Check sheet for the modelled part. Datum: model origin and axes. Units: mm. Round coordinates to 2 decimals unless told otherwise and drop trailing zeros. Loops run counter-clockwise (first coordinate to the right, second up) from the corner with the lowest first, then second, coordinate; pieces in that order, holes last. Notation, with made-up numbers: (85.25, 4) - (142.25, 4) arc R8 cw to (142.25, 15) - close; hole circle Ø4 at (56.25, 74.5). An arc over 180 degrees is marked (long way). Put each result on its own line as item: value. Start each with the question number.
Item 1: Material ranges on line 1 along X through (y, z) = (6, -5); line 2 along X through (y, z) = (9, -41.5); line 3 along Y through (x, z) = (26.75, -26.5), recorded low to high.
Item 2: Section check A-A, the plane z = -11. Record the cut outline in (x, y) (3 decimals).
Item 3: Section check C-C, the plane y = 8.5. Record the cut outline in (x, z), and give its area (3 significant figures).
Item 4: Draft check along X on faces 1 (the flat face through (16, 8, -50.8)), 2 (the cylindrical face through (15.806, 18.283, -25.756)), 3 (the flat face through (25.434, 10.939, -25.044)). Enter one of: pulls with the +X half, pulls with the -X half, needs draft (parallel to the pull), parting line crosses it, or undercut.
Item 5: Gauge pin test, flat ends, axial feed: pin 1 Ø4 at (x, z) = (14, -26.5) entering from +Y; pin 2 Ø1 at (x, z) = (23, -16) entering from +Y; pin 3 Ø5 at (y, z) = (8.5, -36) entering from +X. Record the tip position at first contact, or that the pin passes through.
Item 6: Section check B-B, the plane x = 14. Record the cut outline in (y, z), and give its area (3 significant figures).
from build123d import *

# Parameters (mm, degrees)
SKETCH1_W           = 31.75
SKETCH1_H           = 19.05
BOSS_EXTRUDE1_DEPTH = 50.8
CUT_EXTRUDE1_DEPTH  = 63.861792847
CUT_EXTRUDE2_START  = -50.8
CUT_EXTRUDE2_DEPTH  = 50.8


# Read off the part's stored shape, not the designer's step: Cut-Extrude2
with BuildPart() as part:
    # Sketch1 → Boss-Extrude1 (new body)
    with BuildSketch(Plane.XY):
        with Locations((15.875, 9.525)):
            Rectangle(SKETCH1_W, SKETCH1_H)
    extrude(amount=-BOSS_EXTRUDE1_DEPTH)

    # Sketch2 → Cut-Extrude1 (cut, through all)
    with BuildSketch(Plane.XY):
        Polygon((0, 19.05), (0, 0), (10.998522628, 19.05), align=None)
        Polygon((31.75, 19.05), (31.75, 0), (20.751477372, 19.05), align=None)
    extrude(amount=-CUT_EXTRUDE1_DEPTH, mode=Mode.SUBTRACT)

    # Cut-Extrude2 outline → Cut-Extrude2 (cut)
    with BuildSketch(Plane.XY.offset(CUT_EXTRUDE2_START)):
        with BuildLine():
            Line((20.751477372, 19.05), (10.998522628, 19.05))
            ThreePointArc((10.998522628, 19.05), (15.875, 18.282468135), (20.751477372, 19.05))
        make_face()
        with BuildLine():
            ThreePointArc((15.875, 0), (8.655401308, 0.77169236), (1.762015854, 3.051900982))
            Line((1.762015854, 3.051900982), (0, 0))
            Line((0, 0), (15.875, 0))
        make_face()
        with BuildLine():
            Line((31.75, 0), (29.987984146, 3.051900982))
            ThreePointArc((29.987984146, 3.051900982), (23.094598692, 0.77169236), (15.875, 0))
            Line((15.875, 0), (31.75, 0))
        make_face()
    extrude(amount=CUT_EXTRUDE2_DEPTH, mode=Mode.SUBTRACT)


solid = part.part
Check result:
1. line 1: 3.46 to 28.29
1. line 2: 5.2 to 26.55
1. line 3: 1.78 to 8.66
2. outline: (1.762, 3.052) arc R34.157 ccw to (29.988, 3.052) - (20.751, 19.05) arc R15.875 cw to (10.999, 19.05) - close
3. outline: (4.91, -50.8) - (26.84, -50.8) - (26.84, 0) - (4.91, 0) - close
3. area: 1,110 mm²
4. face 1: needs draft
4. face 2: undercut
4. face 3: pulls with the +X half
5. pin 1: y = 18.76
5. pin 2: y = 16.02
5. pin 3: x = 28.29
6. outline: (0.05, -50.8) - (18.39, -50.8) - (18.39, 0) - (0.05, 0) - close
6. area: 932 mm²
